Verification items for the finished model (mm, model axes). Face numbers are marked on the shaded views. A direction names the side the tool comes from. Round coordinates to 2 decimals unless told otherwise and drop trailing zeros. Write each loop counter-clockwise with the first axis right and the second up, starting at its lowest first coordinate (ties: lowest second). Pieces come first, ordered by that corner, then holes.
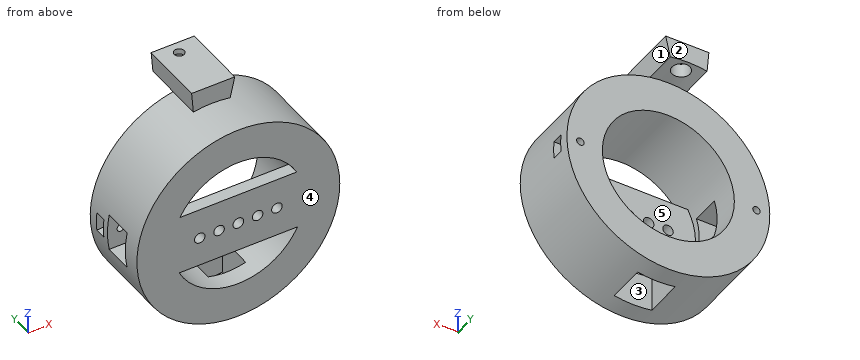
from build123d import *

# Parameters (mm, degrees)
F0_R      = 40.5
F0_R_2    = 26.35
F1_DEPTH  = 30
F3_R      = 1.5
F3_R_2    = 1.4971843494
F4_DEPTH  = 20
F5_DEPTH  = 4.5
F8_R      = 2.1
F9_DEPTH  = 5
F11_DEPTH = 7.5
F13_DEPTH = 7.5
F15_DEPTH = 13
F16_R     = 3.6
F17_DEPTH = 46
F18_R     = 2
F19_DEPTH = 56.1


with BuildPart() as f1:
    # F0 (on Front) → F1 (new body)
    with BuildSketch(Plane.XZ):
        Circle(F0_R)
        Circle(F0_R_2, mode=Mode.SUBTRACT)
    extrude(amount=F1_DEPTH)

    # F3 (on face) → F4 (cut)
    with BuildSketch(Plane(origin=(0, 0, 0), x_dir=(-1, 0, 0), z_dir=(0, 1, 0))):
        with Locations((35.1829901338, 0)):
            Circle(F3_R)
        with Locations((-35.143841058, 0)):
            Circle(F3_R_2)
    extrude(amount=-F4_DEPTH, mode=Mode.SUBTRACT)


with BuildPart() as f5:
    # F2 (on face) → F5 (new body)
    with BuildSketch(Plane(origin=(0, 0, 0), x_dir=(-1, 0, 0), z_dir=(0, 1, 0))):
        with BuildLine():
            Line((31.4417050999, -0.0505083237), (33.2118794322, -3.2991641201))
            Line((33.2118794322, -3.2991641201), (40.3284073856, -3.7241855136))
            ThreePointArc((40.3284073856, -3.7241855136), (40.4570791032, -1.8640682502), (40.5, 0))
            ThreePointArc((40.5, 0), (40.4540427839, 1.9288396616), (40.3162754351, 3.8533018366))
            Line((40.3162754351, 3.8533018366), (33.4046960151, 3.3494916763))
            Line((33.4046960151, 3.3494916763), (31.4417050999, -0.0505083237))
        make_face()
    extrude(amount=-F5_DEPTH)


with BuildPart() as f5b:
    # F2 (on face) → F5, piece 2 (new body)
    with BuildSketch(Plane(origin=(0, 0, 0), x_dir=(-1, 0, 0), z_dir=(0, 1, 0))):
        with BuildLine():
            ThreePointArc((-40.3470564936, 3.5163947881), (-40.499972404, -0.0472787167), (-40.3387366241, -3.6105854882))
            Line((-40.3387366241, -3.6105854882), (-33.3921143039, -3.4494947623))
            Line((-33.3921143039, -3.4494947623), (-31.4291233886, -0.0494947623))
            Line((-31.4291233886, -0.0494947623), (-33.392132321, 3.44931331))
            Line((-33.392132321, 3.44931331), (-40.3470564936, 3.5163947881))
        make_face()
    extrude(amount=-F5_DEPTH)


with BuildPart() as f5_1:
    # F6: moved
    add(f5.part.moved(Location((0, -4, 0))))


with BuildPart() as f5b_1:
    # F6: moved
    add(f5b.part.moved(Location((0, -4, 0))))


with BuildPart() as f1_1:
    add(f1.part)

    # F7: cut F5b, F5
    add(f5b_1.part, mode=Mode.SUBTRACT)
    add(f5_1.part, mode=Mode.SUBTRACT)

    # F8 (on face) → F9 (join)
    with BuildSketch(Plane.XZ.offset(30)):
        with BuildLine():
            Line((23.2959026648, 12.31354616), (-23.2959026648, 12.31354616))
            ThreePointArc((-23.2959026648, 12.31354616), (-26.3476461649, 0.3521953552), (-23.6167164662, -11.68645384))
            Line((-23.6167164662, -11.68645384), (23.6167164662, -11.68645384))
            ThreePointArc((23.6167164662, -11.68645384), (25.6575815197, -6.0009174763), (26.35, 0))
            ThreePointArc((26.35, 0), (25.5750809893, 6.3433218736), (23.2959026648, 12.31354616))
        make_face()
        with Locations((-15.4, 0)):
            Circle(F8_R, mode=Mode.SUBTRACT)
        with BuildLine():
            ThreePointArc((-9.8, 0), (-7.7, 2.1), (-5.6, 0))
            ThreePointArc((-5.6, 0), (-7.7, -2.1), (-9.8, 0))
        make_face(mode=Mode.SUBTRACT)
        with BuildLine():
            ThreePointArc((-2.15, 0), (0, 2.15), (2.15, 0))
            ThreePointArc((2.15, 0), (0, -2.15), (-2.15, 0))
        make_face(mode=Mode.SUBTRACT)
        with BuildLine():
            ThreePointArc((9.8, 0), (7.7, -2.1), (5.6, 0))
            ThreePointArc((5.6, 0), (7.7, 2.1), (9.8, 0))
        make_face(mode=Mode.SUBTRACT)
        with BuildLine():
            ThreePointArc((17.5, 0), (15.4, -2.1), (13.3, 0))
            ThreePointArc((13.3, 0), (15.4, 2.1), (17.5, 0))
        make_face(mode=Mode.SUBTRACT)
    extrude(amount=-F9_DEPTH)

    # F10 (on Right) → F11 (cut, symmetric)
    with BuildSketch(Plane.YZ):
        Polygon((-7.6641152985, -38.8216372541), (-7.6641152985, -23.0135689676), (-22.6641152985, -23.0135689676), (-22.6641152985, -43.0135689676), (-7.6641152985, -43.0135689676), align=None)
    extrude(amount=F11_DEPTH, both=True, mode=Mode.SUBTRACT)

    # F12 (on Top) → F13 (cut, symmetric)
    with BuildSketch(Plane.XY):
        Polygon((-23.9540541172, -11.0713796305), (-43.9540541172, -11.0713796305), (-43.9540541172, -12.5608391675), (-43.9540541172, -22.5713796305), (-23.9540541172, -22.5713796305), align=None)
    extrude(amount=F13_DEPTH, both=True, mode=Mode.SUBTRACT)

    # F14 (on face) → F15 (join, symmetric)
    with BuildSketch(Plane(origin=(0, 0, 0), x_dir=(-1, 0, 0), z_dir=(0, 1, 0))):
        with BuildLine():
            Line((7.388848836, 39.8202826821), (8.0884635863, 48.2109669128))
            Line((8.0884635863, 48.2109669128), (-9.1429123127, 48.1351951361))
            Line((-9.1429123127, 48.1351951361), (-7.3191832289, 39.8331464595))
            ThreePointArc((-7.3191832289, 39.8331464595), (0.0354216515, 40.49998451), (7.388848836, 39.8202826821))
        make_face()
    extrude(amount=F15_DEPTH, both=True)

    # F16 (on Top) → F17 (cut)
    with BuildSketch(Plane.XY):
        with Locations((0, 8.0334944651)):
            Circle(F16_R)
    extrude(amount=F17_DEPTH, mode=Mode.SUBTRACT)

    # F18 (on Top) → F19 (cut)
    with BuildSketch(Plane.XY):
        with Locations((0.0754839784, 8.1013115123)):
            Circle(F18_R)
    extrude(amount=F19_DEPTH, mode=Mode.SUBTRACT)


solid = f1_1.part
Q1. Release check for a two-part mould opening along Z. For the marked faces 1 and 2 record: released by +Z, released by -Z, zero draft, split by the parting line, or undercut.
Recorded:
face 1: undercut
face 2: zero draft
Q2. Sectioned sample at B-B (z = -19). Enter the section's corners in (x, y), plus the area to 3 significant figures.
Recorded:
outline: (-35.77, -30) - (-18.26, -30) - (-18.26, 0) - (-35.77, 0) - close; (18.26, -30) - (35.77, -30) - (35.77, 0) - (18.26, 0) - close
area: 1,050 mm2
Q3. Sectioned sample at D-D (z = 17). Enter the section's corners in (x, y), plus the area to 3 significant figures.
Recorded:
outline: (-36.76, -30) - (-20.13, -30) - (-20.13, 0) - (-36.76, 0) - close; (20.13, -30) - (36.76, -30) - (36.76, 0) - (20.13, 0) - close
area: 998 mm2
Q4. Material ranges on line 1 along Z through (x, y) = (15.4, -28.6); line 2 along Y through (x, z) = (6.5, 5); line 3 along X through (y, z) = (-17.5, -17.5), recorded low to high.
Recorded:
line 1: z = -37.46 to -21.38, -11.69 to -2.1, 2.1 to 12.31, 21.38 to 37.46
line 2: y = -30 to -25
line 3: x = -36.52 to -19.7, 19.7 to 36.52
Q5. Sectioned sample at A-A (x = 0). Give the number of separate pieces and of enclosed holes in the cut face, plus the area to 3 significant figures.
Recorded:
separate pieces: 6
enclosed holes: 0
area: 887 mm2
Q6. Tool access check on the marked faces 3, 4 and 5. Record the directions out of +Z, -Z, +X, -X, +Y, -Y that give a thin tool (end or side, any length) a straight path to the whole face; none if there is none.
Recorded:
face 3: -Z
face 4: +Z, -Z, +X, -X, -Y
face 5: +Y
Q7. Sectioned sample at C-C (x = -15.4). Enter the section's corners in (y, z), plus the area to 3 significant figures.
Recorded:
outline: (-30, -37.46) - (0, -37.46) - (0, -21.38) - (-30, -21.38) - close; (-30, -11.69) - (-25, -11.69) - (-25, -2.1) - (-30, -2.1) - close; (-30, 2.1) - (-25, 2.1) - (-25, 12.31) - (-30, 12.31) - close; (-30, 21.38) - (0, 21.38) - (0, 37.46) - (-30, 37.46) - close
area: 1,060 mm2
Q8. Depth check by flat-ended pin: P1, Ø1, axis at y = -17, z = 33, coming from the +X side; P2, Ø4, axis at x = -5, y = -28, coming from the +Z side; P3, Ø19, axis at x = -1, z = 0, coming from the +Y side; P4, Ø2.5, axis at x = 7.7, z = 0, coming from the -Y side. Enter the tip coordinate at first touch or a pass-through.
Recorded:
P1: stops at x = 24.17
P2: stops at z = 40.39
P3: stops at y = -25
P4: passes through
